```python
from build123d import *

# Parameters (mm, degrees)
SKETCH1_R           = 2.1
BOSS_EXTRUDE1_DEPTH = 500
FILLET1_R           = 0.5


with BuildPart() as part:
    # Sketch1 → Boss-Extrude1 (new body, symmetric)
    with BuildSketch(Plane.XY):
        Polygon((2.839339828, 13.9), (5.5, 16.560660172), (5.5, 18.2), (3.125, 18.2), (3.125, 18.545), (4.58, 20), (10, 20), (10, 14.58), (8.545, 13.125), (8.2, 13.125), (8.2, 15.5), (6.560660172, 15.5), (3.9, 12.839339828), (3.9, 10.2), (3.7, 10), (3.9, 9.8), (3.9, 7.160660172), (6.560660172, 4.5), (8.2, 4.5), (8.2, 6.875), (8.545, 6.875), (10, 5.42), (10, -5.42), (8.545, -6.875), (8.2, -6.875), (8.2, -4.5), (6.560660172, -4.5), (3.9, -7.160660172), (3.9, -9.8), (3.7, -10), (3.9, -10.2), (3.9, -12.839339828), (6.560660172, -15.5), (8.2, -15.5), (8.2, -13.125), (8.545, -13.125), (10, -14.58), (10, -20), (4.58, -20), (3.125, -18.545), (3.125, -18.2), (5.5, -18.2), (5.5, -16.560660172), (2.839339828, -13.9), (0.2, -13.9), (0, -13.7), (-0.2, -13.9), (-2.839339828, -13.9), (-5.5, -16.560660172), (-5.5, -18.2), (-3.125, -18.2), (-3.125, -18.545), (-4.58, -20), (-10, -20), (-10, -14.58), (-8.545, -13.125), (-8.2, -13.125), (-8.2, -15.5), (-6.560660172, -15.5), (-3.9, -12.839339828), (-3.9, -10.2), (-3.7, -10), (-3.9, -9.8), (-3.9, -7.160660172), (-6.560660172, -4.5), (-8.2, -4.5), (-8.2, -6.875), (-8.545, -6.875), (-10, -5.42), (-10, 5.42), (-8.545, 6.875), (-8.2, 6.875), (-8.2, 4.5), (-6.560660172, 4.5), (-3.9, 7.160660172), (-3.9, 9.8), (-3.7, 10), (-3.9, 10.2), (-3.9, 12.839339828), (-6.560660172, 15.5), (-8.2, 15.5), (-8.2, 13.125), (-8.545, 13.125), (-10, 14.58), (-10, 20), (-4.58, 20), (-3.125, 18.545), (-3.125, 18.2), (-5.5, 18.2), (-5.5, 16.560660172), (-2.839339828, 13.9), (-0.2, 13.9), (0, 13.7), (0.2, 13.9), align=None)
        with Locations((0, 10)):
            Circle(SKETCH1_R, mode=Mode.SUBTRACT)
        with Locations((0, -10)):
            Circle(SKETCH1_R, mode=Mode.SUBTRACT)
        Polygon((8.2, -3), (8.2, 3), (5.939339828, 3), (2.839339828, 6.1), (0.2, 6.1), (0, 6.3), (-0.2, 6.1), (-2.839339828, 6.1), (-5.939339828, 3), (-8.2, 3), (-8.2, -3), (-5.939339828, -3), (-2.839339828, -6.1), (-0.2, -6.1), (0, -6.3), (0.2, -6.1), (2.839339828, -6.1), (5.939339828, -3), align=None, mode=Mode.SUBTRACT)
    extrude(amount=BOSS_EXTRUDE1_DEPTH, both=True)

    # Fillet1
    fillet1_edges = [part.edges().sort_by_distance(p)[0] for p in [
        (10, -20, 0),
        (-10, -20, 0),
        (-10, 20, 0),
        (10, 20, 0),
    ]]
    fillet(fillet1_edges, radius=FILLET1_R)


solid = part.part
```
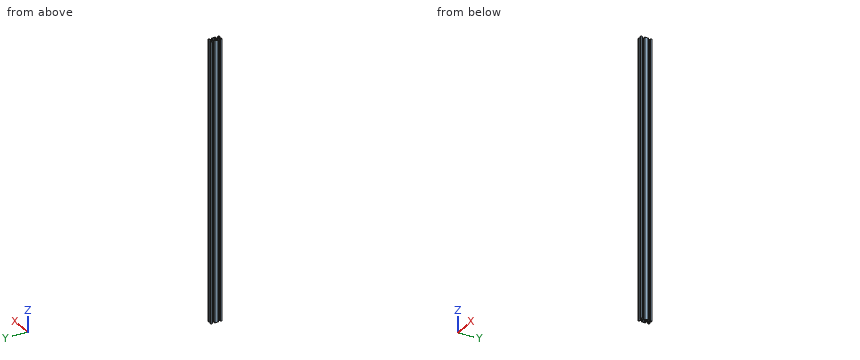
For this review, take the finished solid that the model builds, in its own axes (mm). Round coordinates to 2 decimals unless told otherwise and drop trailing zeros.
1) Insertion check: pin 1 Ø4 at (y, z) = (-12.5, -144) entering from +X; pin 2 Ø3 at (y, z) = (-11.5, -247) entering from +X; pin 3 Ø1 at (x, z) = (0.5, -70.5) entering from -Y. Each pin has a flat end and moves straight along its axis. Give the tip position at first contact, or say it passes through.
Answer below:
pin 1: stops at x = 9.92
pin 2: stops at x = 4.06
pin 3: stops at y = -13.9
2) Take a section at A-A on z = 373. State how many separate pieces and enclosed holes the cut face has, then the cut area to 3 significant figures.
Answer below:
separate pieces: 1
enclosed holes: 3
area: 297 mm2
3) For line 1 along Y through (x, z) = (0, 118.5); line 2 along X through (y, z) = (15, -385); line 3 along X through (y, z) = (0, -449), list the stretches that pass through material, from the lowest coordinate up.
Answer below:
line 1: y = -13.7 to -12.1, -7.9 to -6.3, 6.3 to 7.9, 12.1 to 13.7
line 2: x = -10 to -8.2, -6.06 to -3.94, 3.94 to 6.06, 8.2 to 10
line 3: x = -10 to -8.2, 8.2 to 10
